from build123d import *

# Parameters (mm, degrees)
ESQUISSE1_R        = 11
BOSS_EXTRU_1_DEPTH = 5
D_GAGEMENT_M21_D   = 2.4


with BuildPart() as part:
    # Esquisse1 → Boss.-Extru.1 (new body)
    with BuildSketch(Plane.XY):
        with BuildLine():
            Line((0, 0), (80, 0))
            Line((80, 0), (80, 5))
            Line((80, 5), (70, 5))
            ThreePointArc((70, 5), (62, 13), (70, 21))
            Line((70, 21), (80, 21))
            Line((80, 21), (80, 26))
            Line((80, 26), (0, 26))
            Line((0, 26), (0, 21))
            Line((0, 21), (10, 21))
            ThreePointArc((10, 21), (18, 13), (10, 5))
            Line((10, 5), (0, 5))
            Line((0, 5), (0, 0))
        make_face()
        with Locations((40, 13)):
            Circle(ESQUISSE1_R, mode=Mode.SUBTRACT)
    extrude(amount=BOSS_EXTRU_1_DEPTH)

    # Dégagement M21 (through all)
    with Locations(Plane(origin=(0, 26, 0), x_dir=(1, 0, 0), z_dir=(0, 1, 0))):
        with Locations((76, -2.5), (4, -2.5)):
            Hole(D_GAGEMENT_M21_D / 2)


solid = part.part
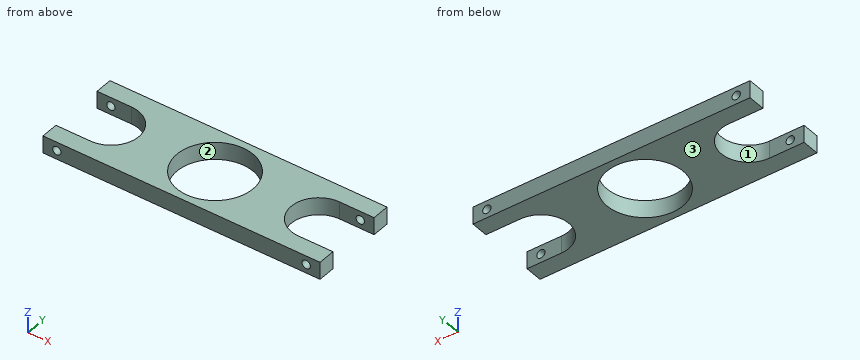
Can you work these out from the model? Positions are in its coordinate system, mm. Face numbers are marked on the shaded views. Coordinates: 2 decimals unless noted, no trailing zeros. Write each loop counter-clockwise with the first axis right and the second up, starting at its lowest first coordinate (ties: lowest second). Pieces come first, ordered by that corner, then holes. Notation, with made-up numbers: (50.25, -8) -> (93.25, -8) arc R11 ccw to (93.25, 3) -> close; hole circle Ø9 at (-18.75, 43). An arc over 180 degrees is marked (long way). Answer as CSV lines item,"result".
1) If we section it at C-C on y = 20: Please give me the cut outline in (x, z), then the cut area to 3 significant figures.
Check result:
outline,"(13.87, 0) -> (31.51, 0) -> (31.51, 5) -> (13.87, 5) -> close; (48.49, 0) -> (66.13, 0) -> (66.13, 5) -> (48.49, 5) -> close"
area,"176 mm²"
2) If we mould it in two halves opening along X, with no side actions, what happens to the marked faces 1, 2 and 3? For each: +X half, -X half, draft (parallel to the pull), parting line (faces both ways), or undercut.
Check result:
face 1,"-X half"
face 2,"undercut"
face 3,"draft"
3) If I drill on line 1 (Z direction, x = 4, y = 22.6); line 2 (Y direction, x = 40, z = 3.5); line 3 (Y direction, x = 7.5, z = 4.8), over which ranges is the centre line in solid material (lowest first)? Write a range as from..to.
Check result:
line 1,"0..1.3, 3.7..5"
line 2,"0..2, 24..26"
line 3,"0..5, 21..26"
4) Will this pin go through, and if not, where does the flat tip stop? P1, Ø1.9, axis at x = 76, z = 2.5, coming from the -Y side.
Check result:
P1,"through"
5) If we section it at B-B on x = 76: Please give me the cut outline in (y, z), then the cut area to 3 significant figures.
Check result:
outline,"(0, 0) -> (5, 0) -> (5, 1.3) -> (0, 1.3) -> close; (0, 3.7) -> (5, 3.7) -> (5, 5) -> (0, 5) -> close; (21, 0) -> (26, 0) -> (26, 1.3) -> (21, 1.3) -> close; (21, 3.7) -> (26, 3.7) -> (26, 5) -> (21, 5) -> close"
area,"26.0 mm²"
6) If we section it at A-A on x = 40: Please give me the cut outline in (y, z).
Check result:
outline,"(0, 0) -> (2, 0) -> (2, 5) -> (0, 5) -> close; (24, 0) -> (26, 0) -> (26, 5) -> (24, 5) -> close"
